Verification items for the finished model (mm, model axes). A direction names the side the tool comes from. Coordinates: 2 decimals unless noted, no trailing zeros. Order: outer loops, then holes, each group sorted by start corner. A loop starts at its lowest first (then second) coordinate and runs counter-clockwise, first axis right, second up. Notation, with made-up numbers: M 25.5,12 L 65.5,12 A34 cw 65.5,48 Z; hole C 30.5,-11.75 d7. An arc over 180 degrees is marked long. Answer as a JSON object with one key per item and string values. Group by question number.
(1) Material ranges on line 1 (Z direction, x = 113.5, y = 9) (3 decimals); line 2 (Z direction, x = 18.5, y = -53.5) (3 decimals); line 3 (X direction, y = -12, z = 19) (3 decimals), recorded low to high.
(2) Access from +Z, -Z, +X, -X, +Y, -Y to the whole of each face (thin tool, end or side, straight path). Record for faces 1 (the face through (52, 25.4, 48)), 2 (the face through (52, -25.4, 48)), 3 (the face through (-3, -7.938, 30)), 4 (the face through (32.088, 16.547, 51.325)), 5 (the face through (41.275, -1, 4)).
(3) Gauge pin test, flat ends, axial feed: pin 1 Ø3 at (x, z) = (33, 46) entering from -Y; pin 2 Ø5 at (y, z) = (48.5, 0) entering from +X (3 decimals); pin 3 Ø1 at (x, y) = (63.5, -11.5) entering from -Z; pin 4 Ø19 at (y, z) = (21, 17.5) entering from -X (3 decimals). Record the tip position at first contact, or that the pin passes through.
(4) Cross-section at A-A (x = 85.5). Enter the section's corners in (y, z) (3 decimals), plus the area to 3 significant figures.
(5) Cross-section at B-B (z = -0.5). Enter the section's corners in (x, y) (3 decimals).
(6) Cross-section at C-C (y = 49.5). Enter the section's corners in (x, z) (3 decimals), plus the area to 3 significant figures.
from build123d import *

# Parameters (mm, degrees)
F1_DEPTH = 63.5
F0_W     = 25.4
F0_H     = 19.05
F2_DEPTH = 25.4
F3_DEPTH = 7.9375


with BuildPart() as f1:
    # F0 (on Front) → F1 (new body, symmetric)
    with BuildSketch(Plane.XZ):
        Polygon((22.225, 9.525), (-41.275, 9.525), (-41.275, -9.525), (41.275, -9.525), (41.275, 9.525), align=None)
    extrude(amount=F1_DEPTH, both=True)

    # F0 (on Front) → F2 (join, symmetric)
    with BuildSketch(Plane.XZ):
        with BuildLine():
            Line((22.225, 27.0002), (22.225, 9.525))
            Line((22.225, 9.525), (41.275, 9.525))
            Line((41.275, 9.525), (41.275, 27.0002))
            ThreePointArc((41.275, 27.0002), (45.92468, 38.22552), (57.15, 42.8752))
            Line((57.15, 42.8752), (74.031852, 42.8752))
            Line((74.031852, 42.8752), (74.031852, 61.9252))
            Line((74.031852, 61.9252), (57.15, 61.9252))
            add(Edge.make_bspline(
                [(55.365015, 61.879556), (55.960003, 61.898055), (56.555027, 61.913281), (57.15, 61.9252)],
                knots=[110.145036, 110.145036, 110.145036, 110.145036, 111.504536, 111.504536, 111.504536, 111.504536], degree=3))
            ThreePointArc((55.365015, 61.879556), (31.831072, 51.05654), (22.225, 27.0002))
        make_face()
        with Locations((86.731852, 52.4002)):
            Rectangle(F0_W, F0_H)
    extrude(amount=F2_DEPTH, both=True)

    # F0 (on Front) → F3 (join, symmetric)
    with BuildSketch(Plane.XZ):
        with BuildLine():
            add(Edge.make_bspline(
                [(-41.275, 9.525), (-40.801804, 37.387647), (7.159855, 60.38073), (55.365015, 61.879556)],
                knots=[0, 0, 0, 0, 110.145036, 110.145036, 110.145036, 110.145036], degree=3))
            Line((-41.275, 9.525), (22.225, 9.525))
            Line((22.225, 9.525), (22.225, 27.0002))
            ThreePointArc((22.225, 27.0002), (31.831072, 51.05654), (55.365015, 61.879556))
        make_face()
    extrude(amount=F3_DEPTH, both=True)

    # F0 (on Front) → F4 (revolve)
    with BuildSketch(Plane.XZ):
        Polygon((99.431852, 66.675), (99.431852, 61.9252), (99.431852, 42.8752), (99.431852, 38.1), (124.831852, 38.1), (124.831852, 66.675), align=None)
    revolve(axis=Axis((99.431852, 0, 52.3875), (0, 0, 1)))


solid = f1.part
Taken from the geometry:
{
 "1": {"line 1": "z = 38.1 to 66.675", "line 2": "z = -9.525 to 9.525", "line 3": "x = 22.225 to 41.275"},
 "2": {"face 1": "+Z, +X, -X, +Y", "face 2": "+Z, +X, -X, -Y", "face 3": "+Z, -X, -Y", "face 4": "+Z, -X, +Y", "face 5": "-Z, +X, +Y, -Y"},
 "3": {"pin 1": "stops at y = -25.4", "pin 2": "stops at x = 41.275", "pin 3": "stops at z = 42.88", "pin 4": "stops at x = -41.275"},
 "4": {"outline": "M -25.4,42.875 L -21.238,42.875 L -21.238,38.1 L 21.238,38.1 L 21.238,42.875 L 25.4,42.875 L 25.4,61.925 L 21.238,61.925 L 21.238,66.675 L -21.238,66.675 L -21.238,61.925 L -25.4,61.925 Z", "area": "1,370 mm²"},
 "5": {"outline": "M -41.275,-63.5 L 41.275,-63.5 L 41.275,63.5 L -41.275,63.5 Z"},
 "6": {"outline": "M -41.275,-9.525 L 41.275,-9.525 L 41.275,9.525 L -41.275,9.525 Z", "area": "1,570 mm²"}
}
